The figure shows three views and two pictorial views of one solid part (mm, origin at its lowest corner). Answer the questions. Give positions to 0.01 mm unless a question says otherwise; leave off trailing zeros. Loops run counter-clockwise (first coordinate to the right, second up) from the corner with the lowest first, then second, coordinate; pieces in that order, holes last.
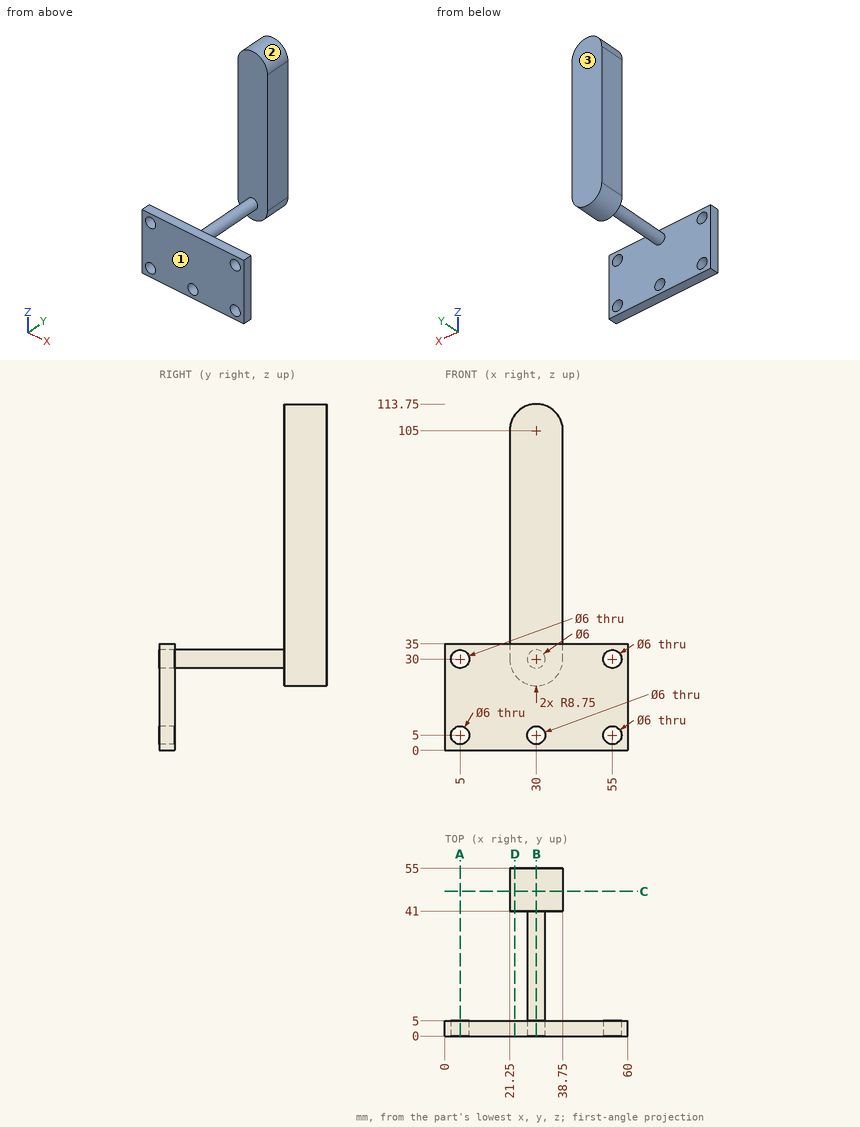
Q1. Section C-C on y = 47.5 is taken. Give the vertices of the cut face in (x, z).
Q2. Section A-A on x = 5 is taken. Give the vertices of the cut face in (y, z).
Q3. Section B-B on x = 30 is taken. Give the vertices of the cut face in (y, z).
Q4. Determine the mould class of the marked faces 1, 2 and 3 for opening direction Y: +Y half, -Y half, draft (parallel to the pull), parting line (faces both ways), or undercut.
Q5. Consider line 1 along X through (y, z) = (3, 30); line 2 along X through (y, z) = (3.75, 5); line 3 along Z through (x, y) = (55, 2.9). Determine where each line is inside the solid, lowest interval first.
Q6. Section D-D on x = 23 is taken. Give the vertices of the cut face in (y, z), plus the area to 3 significant figures.
Q7. Given pin 1 (7 mm diameter, centred on y = 49.5, z = 64, fed in from -X); pin 2 (12 mm diameter, centred on y = 43, z = 22, fed in from +X); pin 3 (9 mm diameter, centred on x = 30.5, z = 86, fed in from -Y); pin 4 (12 mm diameter, centred on x = 19, z = 92.5, fed in from +Y), each flat-ended and moving along its own axis, determine where each tip first touches the part or whether it passes through.
Check result:
1. outline: (21.25, 30) arc R8.75 ccw to (38.75, 30) - (38.75, 105) arc R8.75 ccw to (21.25, 105) - close
2. outline: (0, 0) - (5, 0) - (5, 2) - (0, 2) - close; (0, 8) - (5, 8) - (5, 27) - (0, 27) - close; (0, 33) - (5, 33) - (5, 35) - (0, 35) - close
3. outline: (0, 0) - (5, 0) - (5, 2) - (0, 2) - close; (0, 8) - (5, 8) - (5, 27) - (41, 27) - (41, 21.25) - (55, 21.25) - (55, 113.75) - (41, 113.75) - (41, 33) - (5, 33) - (5, 35) - (0, 35) - close
4. face 1: -Y half
4. face 2: draft
4. face 3: +Y half
5. line 1: x = 0 to 2, 8 to 52, 58 to 60
5. line 2: x = 0 to 2, 8 to 27, 33 to 52, 58 to 60
5. line 3: z = 0 to 2, 8 to 27, 33 to 35
6. outline: (0, 0) - (5, 0) - (5, 35) - (0, 35) - close; (41, 24.75) - (55, 24.75) - (55, 110.25) - (41, 110.25) - close
6. area: 1,370 mm2
7. pin 1: stops at x = 21.25
7. pin 2: stops at x = 38.52
7. pin 3: stops at y = 41
7. pin 4: stops at y = 55
